from build123d import *

# Parameters (mm, degrees)
SKETCH1_R           = 13
SKETCH1_R_2         = 11
BOSS_EXTRUDE1_DEPTH = 90
SKETCH2_R           = 13
BOSS_EXTRUDE2_DEPTH = 5
BOSS_EXTRUDE4_START = 5
SKETCH3_R           = 22
SKETCH3_R_2         = 11
BOSS_EXTRUDE4_DEPTH = 5


with BuildPart() as part:
    # Sketch1 → Boss-Extrude1 (new body)
    with BuildSketch(Plane(origin=(0, 0, 0), x_dir=(0, 0, -1), z_dir=(1, 0, 0))):
        with Locations(Location((0, 0, 0), (0, 0, 180))):
            Circle(SKETCH1_R)
        with Locations(Location((0, 0, 0), (0, 0, 180))):
            Circle(SKETCH1_R_2, mode=Mode.SUBTRACT)
    extrude(amount=BOSS_EXTRUDE1_DEPTH)

    # Sketch2 → Boss-Extrude2 (add)
    with BuildSketch(Plane(origin=(90, 0, 0), x_dir=(0, 0, -1), z_dir=(1, 0, 0))):
        with Locations(Location((0, 0, 0), (0, 0, 180))):
            Circle(SKETCH2_R)
    extrude(amount=BOSS_EXTRUDE2_DEPTH)

    # Sketch3 → Boss-Extrude4 (add)
    with BuildSketch(Plane.ZY.offset(BOSS_EXTRUDE4_START)):
        Circle(SKETCH3_R)
        Circle(SKETCH3_R_2, mode=Mode.SUBTRACT)
    extrude(amount=-BOSS_EXTRUDE4_DEPTH)


solid = part.part
Model file for the job. Use its own axes, mm. A direction names the side the tool comes from. Coordinates: 2 decimals unless noted, no trailing zeros. Loops run counter-clockwise (first coordinate to the right, second up) from the corner with the lowest first, then second, coordinate; pieces in that order, holes last. Notation, with made-up numbers: (-33.75, 37.5) -> (-4.75, 37.5) arc R17 cw to (-4.75, 50.5) -> close; hole circle Ø8 at (0, -10). An arc over 180 degrees is marked (long way). Use one line per item in the form item = value. Start each with the question number.
(1) Cut at B-B on x = 82. Give the cut face in (y, z), and give its area (3 significant figures).
(2) Probe probe 1 along Y at (x, z) = (46, 0); probe 2 along X at (y, z) = (7, -1); probe 3 along X at (y, z) = (-16, 14.5). List the from-to ranges inside material, lowest first. Write a range as from..to.
(3) Tool access for faces 1 (the flat face through (95, 0, 0)), 2 (the cylindrical face through (46.835, 7.91, -10.316)): list every direction of +Z, -Z, +X, -X, +Y, -Y with a clear straight run to the whole face (end or side of a thin tool).
(4) Cut at D-D on z = 12. Give the cut face in (x, y).
(5) Pull direction Z, two halves, no side cores. Call faces 3 (the flat face through (90, 0, 0)), 4 (the cylindrical face through (-2.535, -21.477, -4.769)), 5 (the flat face through (0, -9.5, 9.5)): pulls with the +Z half, pulls with the -Z half, needs draft (parallel to the pull), parting line crosses it, or undercut.
(6) Flat gauge pins, fed straight in: pin 1 (12 mm diameter, centred on x = 57, y = 0.5, fed in from +Z); pin 2 (1.5 mm diameter, centred on x = 60, y = 4.5, fed in from -Z); pin 3 (24 mm diameter, centred on y = 0.5, z = -3.5, fed in from -X); pin 4 (4 mm diameter, centred on x = 55.5, z = 16, fed in from +Y). Where does each tip first touch, or does it go through?
(7) Cut at A-A on y = 0. Give the cut face in (x, z).
Values:
q1.outline = circle Ø26 at (0, 0); hole circle Ø22 at (0, 0)
q1.area = 151 mm2
q2.probe_1 = -13..-11, 11..13
q2.probe_2 = 90..95
q2.probe_3 = -5..0
q3.face_1 = +Z, -Z, +X, +Y, -Y
q3.face_2 = +X
q4.outline = (-5, -18.44) -> (0, -18.44) -> (0, -5) -> (95, -5) -> (95, 5) -> (0, 5) -> (0, 18.44) -> (-5, 18.44) -> close
q5.face_3 = undercut
q5.face_4 = parting line crosses it
q5.face_5 = needs draft
q6.pin_1 = 13
q6.pin_2 = -12.45
q6.pin_3 = -5
q6.pin_4 = through
q7.outline = (-5, -22) -> (0, -22) -> (0, -13) -> (95, -13) -> (95, 13) -> (0, 13) -> (0, 22) -> (-5, 22) -> (-5, 11) -> (90, 11) -> (90, -11) -> (-5, -11) -> close
